from build123d import *

# Parameters (mm, degrees)
BOSS_EXTRUDE1_DEPTH           = 5
BOSS_EXTRUDE1_TAPER           = 2
BOSS_EXTRUDE1_OTHER_WAY_DEPTH = 5
BOSS_EXTRUDE1_OTHER_WAY_TAPER = 2


with BuildPart() as part:
    # Sketch1 → Boss-Extrude1 (new body)
    with BuildSketch(Plane.XY):
        with BuildLine():
            Line((47, 41), (10, 41))
            Line((10, 41), (10, 31))
            ThreePointArc((10, 31), (0, 21), (-10, 31))
            Line((-10, 31), (-10, 41))
            Line((-10, 41), (-47, 41))
            Line((-47, 41), (-57, 31))
            Line((-57, 31), (-57, 12))
            Line((-57, 12), (-43, 12))
            ThreePointArc((-43, 12), (-31, 0), (-43, -12))
            Line((-43, -12), (-57, -12))
            Line((-57, -12), (-57, -31))
            Line((-57, -31), (-47, -41))
            Line((-47, -41), (-10, -41))
            Line((-10, -41), (-10, -31))
            ThreePointArc((-10, -31), (0, -21), (10, -31))
            Line((10, -31), (10, -41))
            Line((10, -41), (47, -41))
            Line((47, -41), (57, -31))
            Line((57, -31), (57, -12))
            Line((57, -12), (43, -12))
            ThreePointArc((43, -12), (31, 0), (43, 12))
            Line((43, 12), (57, 12))
            Line((57, 12), (57, 31))
            Line((57, 31), (47, 41))
        make_face()
    extrude(amount=BOSS_EXTRUDE1_DEPTH, taper=BOSS_EXTRUDE1_TAPER)

    # Sketch1 → Boss-Extrude1 other way (add)
    with BuildSketch(Plane.XY):
        with BuildLine():
            Line((47, 41), (10, 41))
            Line((10, 41), (10, 31))
            ThreePointArc((10, 31), (0, 21), (-10, 31))
            Line((-10, 31), (-10, 41))
            Line((-10, 41), (-47, 41))
            Line((-47, 41), (-57, 31))
            Line((-57, 31), (-57, 12))
            Line((-57, 12), (-43, 12))
            ThreePointArc((-43, 12), (-31, 0), (-43, -12))
            Line((-43, -12), (-57, -12))
            Line((-57, -12), (-57, -31))
            Line((-57, -31), (-47, -41))
            Line((-47, -41), (-10, -41))
            Line((-10, -41), (-10, -31))
            ThreePointArc((-10, -31), (0, -21), (10, -31))
            Line((10, -31), (10, -41))
            Line((10, -41), (47, -41))
            Line((47, -41), (57, -31))
            Line((57, -31), (57, -12))
            Line((57, -12), (43, -12))
            ThreePointArc((43, -12), (31, 0), (43, 12))
            Line((43, 12), (57, 12))
            Line((57, 12), (57, 31))
            Line((57, 31), (47, 41))
        make_face()
    extrude(amount=-BOSS_EXTRUDE1_OTHER_WAY_DEPTH, taper=BOSS_EXTRUDE1_OTHER_WAY_TAPER)


solid = part.part
Geometry: final body of the model. Coordinates: model frame, mm. Give positions to 0.01 mm unless a question says otherwise; leave off trailing zeros. Loops run counter-clockwise (first coordinate to the right, second up) from the corner with the lowest first, then second, coordinate; pieces in that order, holes last. Notation, with made-up numbers: (81.5, 13) - (95.5, 13) arc R20 cw to (95.5, 38) - close; hole circle Ø3 at (-31.5, 7.5). An arc over 180 degrees is marked (long way). Answer as CSV lines item,"result". Start each with the question number.
1. Section B-B, the plane y = 0. Return loops of the section in (x, z).
2. Draft query along Y for faces 1 (the face through (-1, 1, 5)), 2 (the face through (30.914, -0.266, 2.535)), 3 (the face through (0.222, 20.914, -2.535)). Return one class per face: released by +Y, released by -Y, zero draft, split by the parting line, or undercut.
3. Section A-A, the plane x = 0. Return loops of the section in (y, z).
4. Pin query (flat end, axial travel): P1, Ø2, axis at y = 9.5, z = 0, coming from the -X side; P2, Ø4, axis at y = 0, z = -3.5, coming from the -X side; P3, Ø6, axis at y = 27.5, z = 3, coming from the +X side; P4, Ø2, axis at x = 26, z = 2.5, coming from the +Y side. Return the tip coordinate at first contact, or that it passes through.
5. Ray query, L1, parallel to Y at x = -44.5, z = -0.5; L2, parallel to X at y = 17, z = -0.5; L3, parallel to X at y = -29.5, z = -2.5. Return the intervals inside material, ascending.
Answers:
1,outline,"(-31, 0) - (-30.83, -5) - (30.83, -5) - (31, 0) - (30.83, 5) - (-30.83, 5) - close"
2,face 1,"zero draft"
2,face 2,"undercut"
2,face 3,"released by +Y"
3,outline,"(-21, 0) - (-20.83, -5) - (20.83, -5) - (21, 0) - (20.83, 5) - (-20.83, 5) - close"
4,P1,"stops at x = -37.19"
4,P2,"stops at x = -31.05"
4,P3,"stops at x = 57"
4,P4,"stops at y = 40.95"
5,L1,"y = -40.98 to -12.02, 12.02 to 40.98"
5,L2,"x = -56.98 to 56.98"
5,L3,"x = -56.91 to -9.98, 9.98 to 56.91"
